```python
from build123d import *

# Parameters (mm, degrees)
SKETCH1_W                = 83
SKETCH1_H                = 50
BOSS_EXTRUDE1_DEPTH      = 4.7625
SKETCH2_R                = 11
SKETCH2_R_2              = 1.75
CUT_EXTRUDE1_DEPTH       = 98.013820697
CHAMFER1_SIZE            = 5
M5_CLEARANCE_SLOT1_DEPTH = 4.7625


# Read off the part's stored shape, not the designer's step: M5 Clearance Slot1
with BuildPart() as part:
    # Sketch1 → Boss-Extrude1 (new body)
    with BuildSketch(Plane(origin=(0, 0, 0), x_dir=(1, 0, 0), z_dir=(0, 1, 0))):
        with Locations((41.5, 25)):
            Rectangle(SKETCH1_W, SKETCH1_H)
    extrude(amount=BOSS_EXTRUDE1_DEPTH)

    # Sketch2 → Cut-Extrude1 (cut, through all)
    with BuildSketch(Plane(origin=(0, 4.7625, 0), x_dir=(1, 0, 0), z_dir=(0, 1, 0))):
        with Locations(Location((21, 25, 0), (0, 0, 270))):
            Circle(SKETCH2_R)
        with Locations(Location((5.5, 9.5, 0), (0, 0, 270))):
            Circle(SKETCH2_R_2)
        with Locations(Location((36.5, 9.5, 0), (0, 0, 270))):
            Circle(SKETCH2_R_2)
        with Locations(Location((36.5, 40.5, 0), (0, 0, 270))):
            Circle(SKETCH2_R_2)
        with Locations(Location((5.5, 40.5, 0), (0, 0, 270))):
            Circle(SKETCH2_R_2)
    extrude(amount=-CUT_EXTRUDE1_DEPTH, mode=Mode.SUBTRACT)

    # Chamfer1
    chamfer1_edges = [part.edges().sort_by_distance(p)[0] for p in [
        (0, 2.38125, -50),
        (83, 2.38125, -50),
        (83, 2.38125, 0),
        (0, 2.38125, 0),
    ]]
    chamfer(chamfer1_edges, length=CHAMFER1_SIZE)

    # M5 Clearance Slot1 outline → M5 Clearance Slot1 (cut)
    with BuildSketch(Plane(origin=(0, 0, 0), x_dir=(1, 0, 0), z_dir=(0, 1, 0))):
        with BuildLine():
            Line((51.75, 6.75), (56.25, 6.75))
            ThreePointArc((56.25, 6.75), (59, 9.5), (56.25, 12.25))
            Line((56.25, 12.25), (51.75, 12.25))
            ThreePointArc((51.75, 12.25), (49, 9.5), (51.75, 6.75))
        make_face()
        with BuildLine():
            ThreePointArc((76.25, 6.75), (79, 9.5), (76.25, 12.25))
            Line((76.25, 12.25), (71.75, 12.25))
            ThreePointArc((71.75, 12.25), (69, 9.5), (71.75, 6.75))
            Line((71.75, 6.75), (76.25, 6.75))
        make_face()
        with BuildLine():
            Line((71.75, 37.75), (76.25, 37.75))
            ThreePointArc((76.25, 37.75), (79, 40.5), (76.25, 43.25))
            Line((76.25, 43.25), (71.75, 43.25))
            ThreePointArc((71.75, 43.25), (69, 40.5), (71.75, 37.75))
        make_face()
        with BuildLine():
            ThreePointArc((56.25, 37.75), (59, 40.5), (56.25, 43.25))
            Line((56.25, 43.25), (51.75, 43.25))
            ThreePointArc((51.75, 43.25), (49, 40.5), (51.75, 37.75))
            Line((51.75, 37.75), (56.25, 37.75))
        make_face()
    extrude(amount=M5_CLEARANCE_SLOT1_DEPTH, mode=Mode.SUBTRACT)


solid = part.part
```
Input: part model. Units: mm. Frame: model coordinates. A direction names the side the tool comes from. Round coordinates to 2 decimals unless told otherwise and drop trailing zeros. Loops run counter-clockwise (first coordinate to the right, second up) from the corner with the lowest first, then second, coordinate; pieces in that order, holes last. Notation, with made-up numbers: (18.5, 2) -> (30.5, 2) arc R14 ccw to (30.5, 10) -> close; hole circle Ø1 at (72.25, -26.75). An arc over 180 degrees is marked (long way). Use one line per item in the form item = value. Start each with the question number.
Item 1: Section query B-B on z = -15. Return the cut outline in (x, y).
Item 2: Mould query, pull axis Z, two halves, no side actions, for faces 1 (the face through (35.83, 2.415, -7.883)), 2 (the face through (81, 2, -3)), 3 (the face through (41, 2, -50)). Classes: pulls with the +Z half, pulls with the -Z half, needs draft (parallel to the pull), parting line crosses it, or undercut.
Item 3: Section query A-A on x = 36.5. Return the cut outline in (y, z), then the cut area to 3 significant figures.
Item 4: Material intervals for L1, parallel to X at y = 3, z = -9.5; L2, parallel to X at y = 1.65, z = -25; L3, parallel to Z at x = 20.5, y = 1.3, sorted ascending. Write a range as from..to.
Item 5: Contact query for a flat-ended pin moving along its axis: pin 1 Ø3 at (x, z) = (36.5, -9.5) entering from -Y. Output: stop coordinate, or through.
Item 6: Set-up query: faces 4 (the face through (74, 2, -6.75)), 5 (the face through (41, 4.762, -25)). Return all of +Z, -Z, +X, -X, +Y, -Y with unobstructed straight access to the full face (end or side cutting, diameter ignored); none if empty.
Item 7: Section query D-D on x = 21. Return the cut outline in (y, z).
Item 8: Section query C-C on y = 1.4. Count the separate pieces of the cut face and the enclosed holes in it, then the cut area to 3 significant figures.
Ans:
q1.outline = (0, 0) -> (16.42, 0) -> (16.42, 4.76) -> (0, 4.76) -> close; (25.58, 0) -> (83, 0) -> (83, 4.76) -> (25.58, 4.76) -> close
q2.face_1 = undercut
q2.face_2 = pulls with the +Z half
q2.face_3 = pulls with the -Z half
q3.outline = (0, -50) -> (4.76, -50) -> (4.76, -42.25) -> (0, -42.25) -> close; (0, -38.75) -> (4.76, -38.75) -> (4.76, -11.25) -> (0, -11.25) -> close; (0, -7.75) -> (4.76, -7.75) -> (4.76, 0) -> (0, 0) -> close
q3.area = 205 mm^2
q4.L1 = 0..3.75, 7.25..34.75, 38.25..49, 59..69, 79..83
q4.L2 = 0..10, 32..83
q4.L3 = -50..-35.99, -14.01..0
q5.pin_1 = through
q6.face_4 = +Y, -Y
q6.face_5 = +Z, -Z, +X, -X, +Y
q7.outline = (0, -50) -> (4.76, -50) -> (4.76, -36) -> (0, -36) -> close; (0, -14) -> (4.76, -14) -> (4.76, 0) -> (0, 0) -> close
q8.separate_pieces = 1
q8.enclosed_holes = 9
q8.area = 3,490 mm^2
